```python
from build123d import *

# Parameters (mm, degrees)
SKIZZE1_W                                            = 100
SKIZZE1_H                                            = 120
AUFSATZ_LINEAR_AUSTRAGEN1_DEPTH                      = 10
F_15_0_15_DURCHMESSER_BOHRUNG1_D                     = 15
M5_GEWINDEBOHRUNG1_D                                 = 4.2
M5_GEWINDEBOHRUNG1_DEPTH                             = 14
M5_GEWINDEBOHRUNG1_TIP                               = 1.2618073
M4_GEWINDEBOHRUNG1_D                                 = 3.3
M4_GEWINDEBOHRUNG1_DEPTH                             = 11.5
M4_GEWINDEBOHRUNG1_TIP                               = 0.991420021
STIRNSENKUNG_F_R_M5_ZYLINDERSCHRAUBE_MIT_D           = 5.5
STIRNSENKUNG_F_R_M5_ZYLINDERSCHRAUBE_MIT_CBORE_D     = 10
STIRNSENKUNG_F_R_M5_ZYLINDERSCHRAUBE_MIT_CBORE_DEPTH = 5.4
F_4_0_4_DURCHMESSER_BOHRUNG2_D                       = 4


with BuildPart() as part:
    # Skizze1 → Aufsatz-Linear austragen1 (new body)
    with BuildSketch(Plane.XY):
        with Locations((0, 60)):
            Rectangle(SKIZZE1_W, SKIZZE1_H)
    extrude(amount=AUFSATZ_LINEAR_AUSTRAGEN1_DEPTH)

    # Ø15.0 (15) Durchmesser Bohrung1 (through all)
    with Locations(Plane.XY.offset(10)):
        with Locations((0, 105)):
            Hole(F_15_0_15_DURCHMESSER_BOHRUNG1_D / 2)

    # M5 Gewindebohrung1
    with Locations(Plane(origin=(0, 0, 0), x_dir=(-1, 0, 0), z_dir=(0, -1, 0))):
        with Locations((0, -5), (35, -5), (-35, -5)):
            Hole(M5_GEWINDEBOHRUNG1_D / 2, depth=M5_GEWINDEBOHRUNG1_DEPTH)
            with Locations((0, 0, -(M5_GEWINDEBOHRUNG1_DEPTH + M5_GEWINDEBOHRUNG1_TIP / 2))):  # 118° drill point
                Cone(0, M5_GEWINDEBOHRUNG1_D / 2, M5_GEWINDEBOHRUNG1_TIP, mode=Mode.SUBTRACT)

    # M4 Gewindebohrung1
    with Locations(Plane(origin=(0, 120, 0), x_dir=(1, 0, 0), z_dir=(0, 1, 0))):
        with Locations((0, -5)):
            Hole(M4_GEWINDEBOHRUNG1_D / 2, depth=M4_GEWINDEBOHRUNG1_DEPTH)
            with Locations((0, 0, -(M4_GEWINDEBOHRUNG1_DEPTH + M4_GEWINDEBOHRUNG1_TIP / 2))):  # 118° drill point
                Cone(0, M4_GEWINDEBOHRUNG1_D / 2, M4_GEWINDEBOHRUNG1_TIP, mode=Mode.SUBTRACT)

    # Stirnsenkung für M5 Zylinderschraube mit Innensechskant2 (through all)
    with Locations(Plane.XY.offset(10)):
        with Locations((0, 67)):
            CounterBoreHole(STIRNSENKUNG_F_R_M5_ZYLINDERSCHRAUBE_MIT_D / 2, STIRNSENKUNG_F_R_M5_ZYLINDERSCHRAUBE_MIT_CBORE_D / 2, STIRNSENKUNG_F_R_M5_ZYLINDERSCHRAUBE_MIT_CBORE_DEPTH)

    # Ø4.0 (4) Durchmesser Bohrung2 (through all)
    with Locations(Plane.XY.offset(10)):
        with Locations((15, 67), (-15, 67)):
            Hole(F_4_0_4_DURCHMESSER_BOHRUNG2_D / 2)


solid = part.part
```
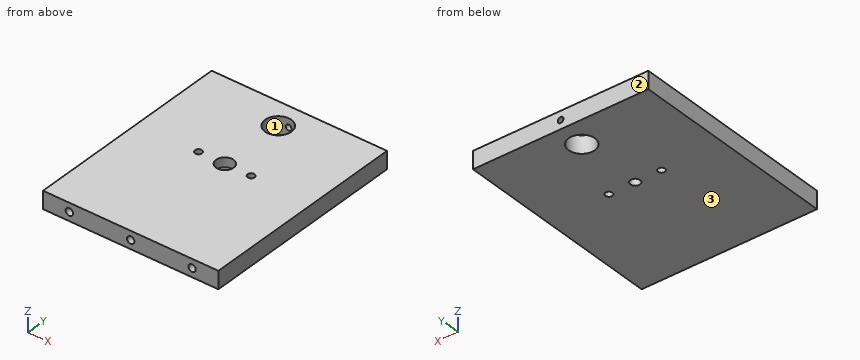
For this review, take the finished solid that the model builds, in its own axes (mm). Face numbers are marked on the shaded views. Give positions to 0.01 mm unless a question says otherwise; leave off trailing zeros. Write each loop counter-clockwise with the first axis right and the second up, starting at its lowest first coordinate (ties: lowest second). Pieces come first, ordered by that corner, then holes.
Item 1: Take a section at B-B (y = 8.5). Give the boundary of the cut face in (x, z), and give its area (3 significant figures).
Item 2: Take a section at A-A (y = 105). Give the boundary of the cut face in (x, z).
Item 3: The part is to be moulded in two halves that separate along Y. For the marked faces 1, 2 and 3, say which applies: +Y half, -Y half, draft (parallel to the pull), parting line (faces both ways), or undercut.
Item 4: Wall thickness on probe 1 along Y at (x, z) = (0, 2.75); probe 2 along Z at (x, y) = (0, 114.25); probe 3 along Y at (x, z) = (15, 7): over which ranges is each line inside the solid? List them lowest first.
Item 5: Insertion check: P1, Ø3.5, axis at x = 0, z = 5, coming from the -Y side; P2, Ø6.5, axis at x = 0, y = 67, coming from the +Z side. Each pin has a flat end and moves straight along its axis. Give the tip position at first contact, or say it passes through.
Established:
1. outline: (-50, 0) - (50, 0) - (50, 10) - (-50, 10) - close; hole circle Ø4.2 at (-35, 5); hole circle Ø4.2 at (0, 5); hole circle Ø4.2 at (35, 5)
1. area: 958 mm2
2. outline: (-50, 0) - (-7.5, 0) - (-7.5, 10) - (-50, 10) - close; (7.5, 0) - (50, 0) - (50, 10) - (7.5, 10) - close
3. face 1: undercut
3. face 2: +Y half
3. face 3: draft
4. probe 1: y = 0 to 64.25, 69.75 to 97.5, 112.5 to 120
4. probe 2: z = 0 to 3.35, 6.65 to 10
4. probe 3: y = 0 to 65, 69 to 120
5. P1: stops at y = 14.21
5. P2: stops at z = 4.6
